from build123d import *

# Parameters (mm, degrees)
SKETCH1_R           = 6.35
SKETCH1_W           = 18.316719234
SKETCH1_H           = 12.7
SKETCH1_W_2         = 17.123051237
BOSS_EXTRUDE1_DEPTH = 19.05
SKETCH2_R           = 12.7
CUT_EXTRUDE1_DEPTH  = 12.7
SKETCH3_R           = 3.175
CUT_EXTRUDE2_DEPTH  = 12.7


with BuildPart() as part:
    # Sketch1 → Boss-Extrude1 (new body)
    # profile 1 of 3: a face of its own
    with BuildSketch(Plane.XY):
        with BuildLine():
            Line((25.4, 25.4), (25.4, 0))
            Line((25.4, 0), (-25.4, 0))
            Line((-25.4, 0), (-25.4, 25.4))
            ThreePointArc((-25.4, 25.4), (0, 50.8), (25.4, 25.4))
        make_face()
        with Locations(Location((0, 25.4, 0), (0, 0, 180))):
            Circle(SKETCH1_R, mode=Mode.SUBTRACT)
    # profile 2 of 3: a face of its own
    with BuildSketch(Plane.XY):
        with Locations((-34.558359617, 6.35)):
            Rectangle(SKETCH1_W, SKETCH1_H)
    # profile 3 of 3: a face of its own
    with BuildSketch(Plane.XY):
        with Locations((33.961525619, 6.35)):
            Rectangle(SKETCH1_W_2, SKETCH1_H)
    extrude(amount=BOSS_EXTRUDE1_DEPTH)

    # Sketch2 → Cut-Extrude1 (cut)
    with BuildSketch(Plane.XY.offset(19.05)):
        with Locations((0, 25.4)):
            Circle(SKETCH2_R)
    extrude(amount=-CUT_EXTRUDE1_DEPTH, mode=Mode.SUBTRACT)

    # Sketch3 → Cut-Extrude2 (cut)
    with BuildSketch(Plane(origin=(0, 12.7, 0), x_dir=(1, 0, 0), z_dir=(0, 1, 0))):
        with Locations(Location((-34.558359617, -9.525, 0), (0, 0, 270))):
            Circle(SKETCH3_R)
        with Locations(Location((33.961525618, -9.525, 0), (0, 0, 270))):
            Circle(SKETCH3_R)
    extrude(amount=-CUT_EXTRUDE2_DEPTH, mode=Mode.SUBTRACT)


solid = part.part
Read the model definition and answer for the solid it produces. Units are mm, in the model's axes. A direction names the side the tool comes from. Round coordinates to 2 decimals unless told otherwise and drop trailing zeros. Write each loop counter-clockwise with the first axis right and the second up, starting at its lowest first coordinate (ties: lowest second). Pieces come first, ordered by that corner, then holes. Notation, with made-up numbers: (10.5, 76.25) - (17.5, 76.25) arc R25 ccw to (17.5, 98.25) - close; hole circle Ø9 at (29.5, -4.75). An arc over 180 degrees is marked (long way). One line per question, with ' | ' between items. Start each with the question number.
1. Section B-B (z = 5.25) is taken. Determine the outline of the cut face in (x, y), and give its area (3 significant figures).
2. Find the intervals of material crossed by probe 1 along X at (y, z) = (26, 17.5); probe 2 along Y at (x, z) = (0, 4); probe 3 along Y at (x, z) = (37, 14.5), in increasing order. Write a range as [from, to].
3. Section A-A (x = 0) is taken. Determine the outline of the cut face in (y, z).
4. Section D-D (y = 35.5) is taken. Determine the outline of the cut face in (x, z), and give its area (3 significant figures).
5. Section C-C (z = 10.75) is taken. Determine the outline of the cut face in (x, y).
6. For faces 1 (the face through (1.38, 31.6, 3.13)), 2 (the face through (-3, 31.2, 6.35)), 3 (the face through (38, 12.7, 9)), determine the directions among +Z, -Z, +X, -X, +Y, -Y from which every point of the face is accessible in a straight line to the end or side of a thin tool.
7. Each of these flat-tipped pins is pushed along its axis until it touches: pin 1 (1.5 mm diameter, centred on x = -20.5, y = 29, fed in from -Z); pin 2 (20.5 mm diameter, centred on x = 0, y = 25.4, fed in from +Z); pin 3 (10 mm diameter, centred on y = 18, z = 5, fed in from -X); pin 4 (2 mm diameter, centred on x = -21.5, z = 16.5, fed in from +Y). Where does it stop, or does it pass through?
8. For a pull along Y with two mould halves and no side action, classify faces 4 (the face through (-25.4, 19, 9)), 5 (the face through (-31, 12.7, 9)), 6 (the face through (6.827, 36.109, 12.789)) as +Y half, -Y half, draft (parallel to the pull), parting line (faces both ways), or undercut.
Filled in:
1) outline: (-43.72, 0) - (42.52, 0) - (42.52, 12.7) - (25.4, 12.7) - (25.4, 25.4) arc R25.4 ccw to (-25.4, 25.4) - (-25.4, 12.7) - (-43.72, 12.7) - close; hole circle Ø12.7 at (0, 25.4) | area: 2,630 mm²
2) probe 1: [-25.39, -12.69], [12.69, 25.39] | probe 2: [0, 19.05], [31.75, 50.8] | probe 3: [0, 12.7]
3) outline: (0, 0) - (19.05, 0) - (19.05, 6.35) - (12.7, 6.35) - (12.7, 19.05) - (0, 19.05) - close; (31.75, 0) - (50.8, 0) - (50.8, 19.05) - (38.1, 19.05) - (38.1, 6.35) - (31.75, 6.35) - close
4) outline: (-23.31, 0) - (23.31, 0) - (23.31, 19.05) - (7.7, 19.05) - (7.7, 6.35) - (-7.7, 6.35) - (-7.7, 19.05) - (-23.31, 19.05) - close | area: 692 mm²
5) outline: (-43.72, 0) - (-37.49, 0) - (-37.49, 12.7) - (-43.72, 12.7) - close; (-31.63, 0) - (31.03, 0) - (31.03, 12.7) - (25.4, 12.7) - (25.4, 25.4) arc R25.4 ccw to (-25.4, 25.4) - (-25.4, 12.7) - (-31.63, 12.7) - close; (36.89, 0) - (42.52, 0) - (42.52, 12.7) - (36.89, 12.7) - close; hole circle Ø25.4 at (0, 25.4)
6) face 1: +Z, -Z | face 2: +Z | face 3: +Z, -Z, +X, +Y
7) pin 1: z = 0 | pin 2: z = 6.35 | pin 3: x = -25.4 | pin 4: y = 40.4
8) face 4: draft | face 5: +Y half | face 6: undercut
